from build123d import *

# Parameters (mm, degrees)
SCHIZZO1_R                   = 3
SCHIZZO1_R_2                 = 4
ESTRUSIONE_ESTRUSIONE1_DEPTH = 54
SCHIZZO2_W                   = 30
SCHIZZO2_H                   = 25
TAGLIO_ESTRUSIONE1_DEPTH     = 34
SMUSSO1_SIZE                 = 5
SMUSSO2_SIZE                 = 10


with BuildPart() as part:
    # Schizzo1 → Estrusione-Estrusione1 (new body)
    with BuildSketch(Plane.XY):
        with BuildLine():
            Line((-48.625413912, -12.5), (75, -12.5))
            Line((75, -12.5), (75, 12.5))
            Line((75, 12.5), (-75, 12.5))
            Line((-75, 12.5), (-75, -12.5))
            ThreePointArc((-75, -12.5), (-70.470091926, -19.386839185), (-62.352385612, -17.954545455))
            ThreePointArc((-62.352385612, -17.954545455), (-56.010903371, -13.913592454), (-48.625413912, -12.5))
        make_face()
        with Locations((63, 0)):
            Circle(SCHIZZO1_R, mode=Mode.SUBTRACT)
        with Locations((17, 0)):
            Circle(SCHIZZO1_R_2, mode=Mode.SUBTRACT)
    extrude(amount=ESTRUSIONE_ESTRUSIONE1_DEPTH)

    # Schizzo2 → Taglio-Estrusione1 (cut)
    with BuildSketch(Plane(origin=(75, 0, 0), x_dir=(0, 0, -1), z_dir=(1, 0, 0))):
        with Locations((-27, 0)):
            Rectangle(SCHIZZO2_W, SCHIZZO2_H)
    extrude(amount=-TAGLIO_ESTRUSIONE1_DEPTH, mode=Mode.SUBTRACT)

    # Smusso1
    smusso1_edges = [part.edges().sort_by_distance(p)[0] for p in [
        (75, -12.5, 48),
        (75, 12.5, 48),
        (75, -12.5, 6),
        (75, 12.5, 6),
    ]]
    chamfer(smusso1_edges, length=SMUSSO1_SIZE)

    # Smusso2
    smusso2_edges = [part.edges().sort_by_distance(p)[0] for p in [
        (-75, 12.5, 27),
    ]]
    chamfer(smusso2_edges, length=SMUSSO2_SIZE)


solid = part.part
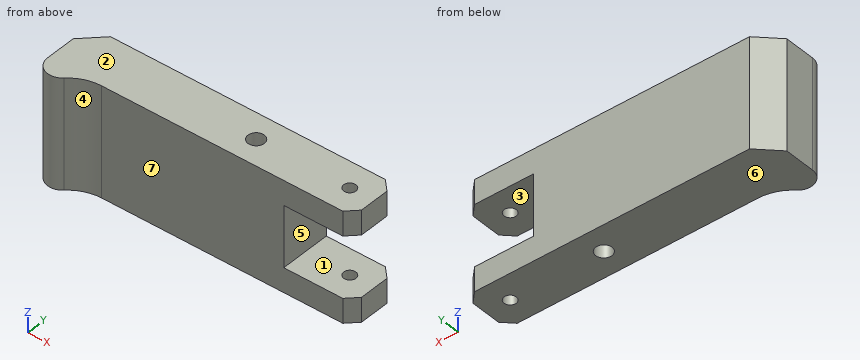
Work out the finished part from the listing and answer in its coordinate system (mm). Face numbers are marked on the shaded views. A direction names the side the tool comes from. Round coordinates to 2 decimals unless told otherwise and drop trailing zeros. Write each loop counter-clockwise with the first axis right and the second up, starting at its lowest first coordinate (ties: lowest second). Pieces come first, ordered by that corner, then holes.
1) Given pin 1 Ø3 at (y, z) = (4.5, 28.5) entering from +X; pin 2 Ø2 at (x, z) = (28.5, 40.5) entering from -Y; pin 3 Ø5 at (x, y) = (63, 0) entering from -Z, each flat-ended and moving along its own axis, determine where each tip first touches the part or whether it passes through.
2) A cutting plane is placed at A-A (z = 7.5). Give the vertices of the cut face in (x, y).
3) A tool of negligible diameter and unlimited length cuts with its end or side. For the marked faces 5, 6 and 7, from which of +Z, -Z, +X, -X, +Y, -Y can it reach the whole face along a straight path? Write none if from no direction.
4) A cutting plane is placed at D-D (x = 17). Give the vertices of the cut face in (y, z), plus the area to 3 significant figures.
5) Straight lines are drawn through the part: line 1 (Y direction, x = 17, z = 17); line 2 (Y direction, x = 63, z = 49.75); line 3 (Z direction, x = 45, y = -1). For each, find the intervals that lie inside material, in ascending order.
6) The mould has two halves that part along Z. Classify the marked faces 1, 2, 3 and 4: pulls with the +Z half, pulls with the -Z half, needs draft (parallel to the pull), parting line crosses it, or undercut.
7) A cutting plane is placed at C-C (y = 0). Give the vertices of the cut face in (x, z), plus the area to 3 significant figures.
8) A cutting plane is placed at B-B (x = 63). Give the vertices of the cut face in (y, z).
Completed:
1. pin 1: stops at x = 41
1. pin 2: stops at y = -12.5
1. pin 3: passes through
2. outline: (-75, -12.5) arc R7.5 ccw to (-62.35, -17.95) arc R20 cw to (-48.63, -12.5) - (70, -12.5) - (75, -7.5) - (75, 7.5) - (70, 12.5) - (-65, 12.5) - (-75, 2.5) - close; hole circle Ø8 at (17, 0); hole circle Ø6 at (63, 0)
3. face 5: +X, +Y, -Y
3. face 6: -Z, +X, -X, +Y, -Y
3. face 7: +Z, -Z, +X, -Y
4. outline: (-12.5, 0) - (-4, 0) - (-4, 54) - (-12.5, 54) - close; (4, 0) - (12.5, 0) - (12.5, 54) - (4, 54) - close
4. area: 918 mm2
5. line 1: y = -12.5 to -4, 4 to 12.5
5. line 2: y = -12.5 to -3, 3 to 12.5
5. line 3: z = 0 to 12, 42 to 54
6. face 1: undercut
6. face 2: pulls with the +Z half
6. face 3: undercut
6. face 4: needs draft
7. outline: (-75, 0) - (13, 0) - (13, 54) - (-75, 54) - close; (21, 0) - (60, 0) - (60, 12) - (41, 12) - (41, 42) - (60, 42) - (60, 54) - (21, 54) - close; (66, 0) - (75, 0) - (75, 12) - (66, 12) - close; (66, 42) - (75, 42) - (75, 54) - (66, 54) - close
7. area: 6,500 mm2
8. outline: (-12.5, 0) - (-3, 0) - (-3, 12) - (-12.5, 12) - close; (-12.5, 42) - (-3, 42) - (-3, 54) - (-12.5, 54) - close; (3, 0) - (12.5, 0) - (12.5, 12) - (3, 12) - close; (3, 42) - (12.5, 42) - (12.5, 54) - (3, 54) - close
